Work out the finished part from the listing and answer in its coordinate system (mm). Face numbers are marked on the shaded views. Give positions to 0.01 mm unless a question says otherwise; leave off trailing zeros. Write each loop counter-clockwise with the first axis right and the second up, starting at its lowest first coordinate (ties: lowest second). Pieces come first, ordered by that corner, then holes. Notation, with made-up numbers: (47, 31.25) -> (59, 31.25) arc R16 cw to (59, 41.25) -> close; hole circle Ø11 at (-37, 58). An arc over 180 degrees is marked (long way). Use a Markdown table: item, result. Add a question column.
Q1. Consider line 1 (Y direction, x = 0, z = 1.85); line 2 (X direction, y = 8, z = 0.95); line 3 (X direction, y = -2, z = 2.4). Determine where each line is inside the solid, lowest interval first.
Q2. Section B-B, the plane y = 21 is taken. Give the vertices of the cut face in (x, z).
Q3. Section D-D, the plane x = -7 is taken. Give the vertices of the cut face in (y, z), plus the area to 3 significant figures.
Q4. Section C-C, the plane z = 0.55 is taken. Give the vertices of the cut face in (x, y), plus the area to 3 significant figures.
Q5. Each of these flat-tipped pins is pushed along its axis until it touches: pin 1 Ø3.5 at (x, y) = (0, 20) entering from +Z; pin 2 Ø1.5 at (y, z) = (18.5, 1) entering from -X; pin 3 Ø1.5 at (x, z) = (1, 1) entering from -Y; pin 4 Ø1 at (x, z) = (-16, 0.5) entering from +Y. Where does it stop, or does it pass through?
Q6. For a pull along Y with two mould halves and no side action, classify the marked faces 1, 2, 3 and 4 as pulls with the +Y half, pulls with the -Y half, needs draft (parallel to the pull), parting line crosses it, or undercut.
Q7. Section A-A, the plane x = 0 is taken. Give the vertices of the cut face in (y, z), plus the area to 3 significant figures.
from build123d import *

# Parameters (mm, degrees)
SKETCH1_R           = 3
SKETCH1_R_2         = 2.5
BOSS_EXTRUDE1_DEPTH = 3
FILLET1_R           = 20


with BuildPart() as part:
    # Sketch1 → Boss-Extrude1 (new body)
    with BuildSketch(Plane.XY):
        with BuildLine():
            Line((-8, 0), (-8, 17.856406461))
            Line((-8, 17.856406461), (-19.692234478, 38.107950631))
            ThreePointArc((-19.692234478, 38.107950631), (-16.764031248, 49.036153861), (-5.835828018, 46.107950631))
            Line((-5.835828018, 46.107950631), (8, 22.143593539))
            Line((8, 22.143593539), (8, 0))
            ThreePointArc((8, 0), (0, -8), (-8, 0))
        make_face()
        Circle(SKETCH1_R, mode=Mode.SUBTRACT)
        with Locations((0, 20)):
            Circle(SKETCH1_R, mode=Mode.SUBTRACT)
        with Locations((-12.749783974, 42.112266724)):
            Circle(SKETCH1_R_2, mode=Mode.SUBTRACT)
    extrude(amount=BOSS_EXTRUDE1_DEPTH)

    # Fillet1
    fillet1_edges = [part.edges().sort_by_distance(p)[0] for p in [
        (-8, 17.856406461, 1.5),
        (8, 22.143593539, 1.5),
    ]]
    fillet(fillet1_edges, radius=FILLET1_R)


solid = part.part
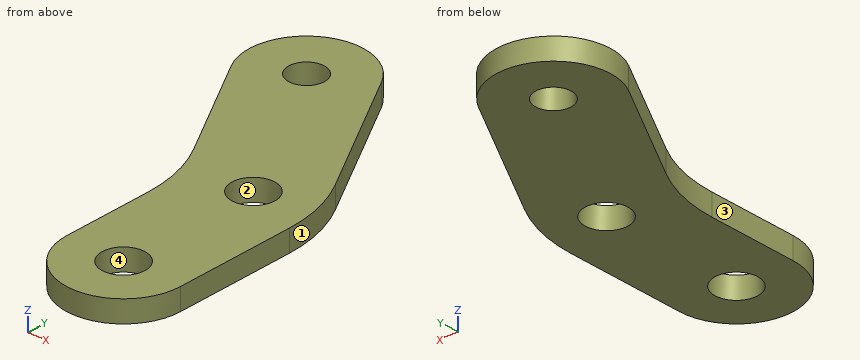
Result set:
| question | item | result |
|---|---|---|
| 1 | line 1 | y = -8 to -3, 3 to 17, 23 to 36 |
| 1 | line 2 | x = -8 to 8 |
| 1 | line 3 | x = -7.75 to -2.24, 2.24 to 7.75 |
| 2 | outline | (-9.9, 0) -> (-2.83, 0) -> (-2.83, 3) -> (-9.9, 3) -> close; (2.83, 0) -> (7.55, 0) -> (7.55, 3) -> (2.83, 3) -> close |
| 3 | outline | (-3.87, 0) -> (47.66, 0) -> (47.66, 3) -> (-3.87, 3) -> close |
| 3 | area | 155 mm2 |
| 4 | outline | (-19.69, 38.11) -> (-10.68, 22.5) arc R20 cw to (-8, 12.5) -> (-8, 0) arc R8 ccw to (8, 0) -> (8, 16.78) arc R20 ccw to (5.32, 26.78) -> (-5.84, 46.11) arc R8 ccw to start; hole circle Ø5 at (-12.75, 42.11); hole circle Ø6 at (0, 0); hole circle Ø6 at (0, 20) |
| 4 | area | 853 mm2 |
| 5 | pin 1 | passes through |
| 5 | pin 2 | stops at x = -9.17 |
| 5 | pin 3 | stops at y = -8 |
| 5 | pin 4 | stops at y = 49.63 |
| 6 | face 1 | pulls with the +Y half |
| 6 | face 2 | undercut |
| 6 | face 3 | needs draft |
| 6 | face 4 | undercut |
| 7 | outline | (-8, 0) -> (-3, 0) -> (-3, 3) -> (-8, 3) -> close; (3, 0) -> (17, 0) -> (17, 3) -> (3, 3) -> close; (23, 0) -> (36, 0) -> (36, 3) -> (23, 3) -> close |
| 7 | area | 96.0 mm2 |
